from build123d import *

# Parameters (mm, degrees)
BOSS_EXTRUDE1_DEPTH = 5
SKETCH2_W           = 200
SKETCH2_H           = 5
BOSS_EXTRUDE2_DEPTH = 15
BOSS_EXTRUDE3_DEPTH = 15
SKETCH6_R           = 2.15
CUT_EXTRUDE2_DEPTH  = 175.212513902
CUT_EXTRUDE3_DEPTH  = 3.2
SKETCH9_W           = 20
SKETCH9_H           = 11
BOSS_EXTRUDE4_DEPTH = 2
CHAMFER1_SIZE       = 2
CUT_EXTRUDE4_DEPTH  = 175.051716452
CUT_EXTRUDE5_DEPTH  = 175.212513902
BOSS_EXTRUDE5_START = 6
BOSS_EXTRUDE5_DEPTH = 6
FILLET1_R           = 2


with BuildPart() as part:
    # Sketch1 → Boss-Extrude1 (new body)
    with BuildSketch(Plane(origin=(0, 0, 0), x_dir=(1, 0, 0), z_dir=(0, 1, 0))):
        with BuildLine():
            Line((-100, 0), (100, 0))
            Line((100, 0), (100, 38.1))
            Line((100, 38.1), (-100, 115))
            Line((-100, 115), (-130, 115))
            Line((-130, 115), (-130, 20))
            Line((-130, 20), (-110, 20))
            ThreePointArc((-110, 20), (-102.928932188, 17.071067812), (-100, 10))
            Line((-100, 10), (-100, 0))
        make_face()
    extrude(amount=BOSS_EXTRUDE1_DEPTH)

    # Sketch2 → Boss-Extrude2 (add)
    with BuildSketch(Plane.XZ):
        with Locations((0, -2.5)):
            Rectangle(SKETCH2_W, SKETCH2_H)
    extrude(amount=BOSS_EXTRUDE2_DEPTH)

    # Sketch5 → Boss-Extrude3 (add)
    with BuildSketch(Plane.XZ):
        Polygon((-53.5, -5), (-34.5, -5), (-39.5, -10), (-48.5, -10), align=None)
        Polygon((68.5, -10), (77.5, -10), (82.5, -5), (63.5, -5), align=None)
    extrude(amount=BOSS_EXTRUDE3_DEPTH)

    # Sketch6 → Cut-Extrude2 (cut, through all)
    with BuildSketch(Plane.XY):
        with Locations((-44, -7)):
            Circle(SKETCH6_R)
        with Locations((73, -7)):
            Circle(SKETCH6_R)
    extrude(amount=-CUT_EXTRUDE2_DEPTH, mode=Mode.SUBTRACT)

    # Sketch7 → Cut-Extrude3 (cut)
    with BuildSketch(Plane(origin=(0, 0, -10), x_dir=(-1, 0, 0), z_dir=(0, 0, -1))):
        Polygon((-73, -11.099186911), (-69.45, -9.049593456), (-69.45, -4.950406544), (-73, -2.900813089), (-76.55, -4.950406544), (-76.55, -9.049593456), align=None)
        Polygon((47.55, -9.049593456), (47.55, -4.950406544), (44, -2.900813089), (40.45, -4.950406544), (40.45, -9.049593456), (44, -11.099186911), align=None)
    extrude(amount=-CUT_EXTRUDE3_DEPTH, mode=Mode.SUBTRACT)

    # Sketch9 → Boss-Extrude4 (add)
    with BuildSketch(Plane.XZ):
        with Locations((-115, -30)):
            Rectangle(SKETCH9_W, SKETCH9_H)
        with Locations((-115, -105)):
            Rectangle(SKETCH9_W, SKETCH9_H)
    extrude(amount=BOSS_EXTRUDE4_DEPTH)

    # Chamfer1
    chamfer1_edges = [part.edges().sort_by_distance(p)[0] for p in [
        (-105, 0, -30),
        (-115, 0, -35.5),
        (-115, 0, -24.5),
        (-125, 0, -30),
        (-115, 0, -99.5),
        (-125, 0, -105),
        (-105, 0, -105),
        (-115, 0, -110.5),
    ]]
    chamfer(chamfer1_edges, length=CHAMFER1_SIZE - 0.0001)  # a hair under: the kernel refuses the full size

    # Sketch8 → Cut-Extrude4 (cut, through all)
    with BuildSketch(Plane.XZ.offset(2)):
        with BuildLine():
            Line((-118, -27.95), (-112, -27.95))
            ThreePointArc((-112, -27.95), (-109.95, -30), (-112, -32.05))
            Line((-112, -32.05), (-118, -32.05))
            ThreePointArc((-118, -32.05), (-120.05, -30), (-118, -27.95))
        make_face()
        with BuildLine():
            Line((-118, -102.95), (-112, -102.95))
            ThreePointArc((-112, -102.95), (-109.95, -105), (-112, -107.05))
            Line((-112, -107.05), (-118, -107.05))
            ThreePointArc((-118, -107.05), (-120.05, -105), (-118, -102.95))
        make_face()
    extrude(amount=-CUT_EXTRUDE4_DEPTH, mode=Mode.SUBTRACT)

    # Sketch10 → Cut-Extrude5 (cut, through all)
    with BuildSketch(Plane.XZ):
        with BuildLine():
            Line((-90, -31.398310884), (-90, -85.359919445))
            ThreePointArc((-90, -85.359919445), (-88.698533585, -87.832768745), (-85.923344225, -88.160064502))
            Line((-85.923344225, -88.160064502), (63.076655775, -30.869564502))
            ThreePointArc((63.076655775, -30.869564502), (64.4728493, -29.76795303), (65, -28.069419445))
            Line((65, -28.069419445), (65, -23))
            ThreePointArc((65, -23), (64.121320344, -20.878679656), (62, -20))
            Line((62, -20), (-87, -20))
            ThreePointArc((-87, -20), (-89.121320344, -20.878679656), (-90, -23))
            Line((-90, -23), (-90, -31.398310884))
        make_face()
    extrude(amount=-CUT_EXTRUDE5_DEPTH, mode=Mode.SUBTRACT)

    # Sketch11 → Boss-Extrude5 (add)
    with BuildSketch(Plane.XZ.offset(BOSS_EXTRUDE5_START)):
        with BuildLine():
            Line((62, -17.75), (-87, -17.75))
            ThreePointArc((-87, -17.75), (-90.712310601, -19.287689399), (-92.25, -23))
            Line((-92.25, -23), (-92.25, -85.359919445))
            ThreePointArc((-92.25, -85.359919445), (-89.972433773, -89.68740572), (-85.115852394, -90.260173296))
            Line((-85.115852394, -90.260173296), (63.884147606, -32.969673296))
            ThreePointArc((63.884147606, -32.969673296), (66.327486275, -31.041853218), (67.25, -28.069419445))
            Line((67.25, -28.069419445), (67.25, -23))
            ThreePointArc((67.25, -23), (65.712310601, -19.287689399), (62, -17.75))
        make_face()
        with BuildLine():
            Line((-90, -23), (-90, -85.359919445))
            ThreePointArc((-90, -85.359919445), (-88.698533585, -87.832768745), (-85.923344225, -88.160064502))
            Line((-85.923344225, -88.160064502), (63.076655775, -30.869564502))
            ThreePointArc((63.076655775, -30.869564502), (64.4728493, -29.76795303), (65, -28.069419445))
            Line((65, -28.069419445), (65, -23))
            ThreePointArc((65, -23), (64.121320344, -20.878679656), (62, -20))
            Line((62, -20), (-87, -20))
            ThreePointArc((-87, -20), (-89.121320344, -20.878679656), (-90, -23))
        make_face(mode=Mode.SUBTRACT)
    extrude(amount=-BOSS_EXTRUDE5_DEPTH)

    # Fillet1
    fillet1_edges = [part.edges().sort_by_distance(p)[0] for p in [
        (-130, 2.5, -115),
        (-130, 2.5, -20),
        (100, 2.5, -38.1),
        (-100, 2.5, -115),
    ]]
    fillet(fillet1_edges, radius=FILLET1_R)


solid = part.part
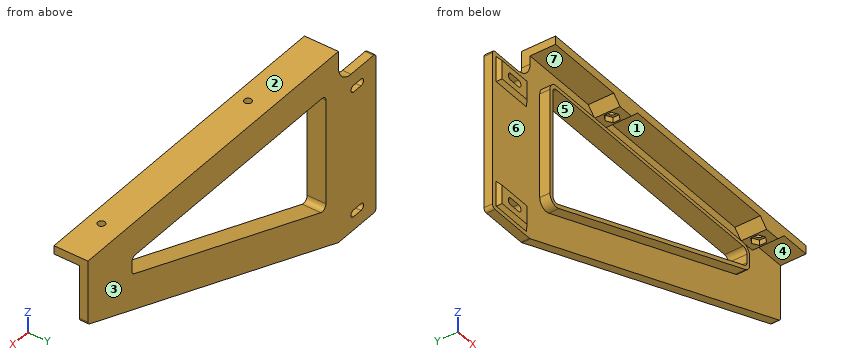
Verification items for the finished model (mm, model axes). Face numbers are marked on the shaded views. A direction names the side the tool comes from. Coordinates: 2 decimals unless noted, no trailing zeros. Order: outer loops, then holes, each group sorted by start corner. A loop starts at its lowest first (then second) coordinate and runs counter-clockwise, first axis right, second up.
Item 1: Section check A-A, the plane z = -74.5. Enter the section's corners in (x, y), then the cut area to 3 significant figures.
Filled in:
outline: (-130, 0) - (-92.25, 0) - (-92.25, -6) - (-90, -6) - (-90, 5) - (-130, 5) - close; (-50.4, -6) - (-44.13, -6) - (-44.13, 0) - (5.33, 0) - (5.33, 5) - (-50.4, 5) - close
area: 530 mm2
Item 2: Access from +Z, -Z, +X, -X, +Y, -Y to the whole of each face (thin tool, end or side, straight path). Record for the marked faces 3, 4, 5, 6 and 7.
Filled in:
face 3: +Z, -Z, +X, -X, +Y
face 4: -Z, +X, -Y
face 5: +Y, -Y
face 6: -Y
face 7: -X, -Y
Item 3: Depth check by flat-ended pin: pin 1 (12 mm diameter, centred on x = -35, z = -67, fed in from -Y); pin 2 (5.5 mm diameter, centred on x = -15, y = -3, fed in from -Z); pin 3 (1.6 mm diameter, centred on y = -7, z = -9, fed in from +X). Enter the tip coordinate at first touch or a pass-through.
Filled in:
pin 1: stops at y = -6
pin 2: stops at z = -64.36
pin 3: stops at x = 79.3
Item 4: Release check for a two-part mould opening along X. For the marked faces 1 and 2 record: +X half, -X half, draft (parallel to the pull), parting line (faces both ways), or undercut.
Filled in:
face 1: undercut
face 2: draft
Item 5: Material ranges on L1, parallel to Y at x = -44, z = -3; L2, parallel to X at y = -9, z = -8.5; L3, parallel to Z at x = 56, y = -1, recorded low to high.
Filled in:
L1: y = -15 to -9.15, -4.85 to 5
L2: x = -50 to -47.55, -40.45 to -38, 67 to 69.45, 76.55 to 79
L3: z = -36 to -33.59, -20 to -17.75, -5 to 0
Item 6: Section check B-B, the plane x = -17. Enter the section's corners in (y, z), then the cut area to 3 significant figures.
Filled in:
outline: (-15, -5) - (0, -5) - (0, -17.75) - (-6, -17.75) - (-6, -20) - (5, -20) - (5, 0) - (-15, 0) - close; (-6, -64.07) - (0, -64.07) - (0, -83.09) - (5, -83.09) - (5, -61.66) - (-6, -61.66) - close
area: 310 mm2
